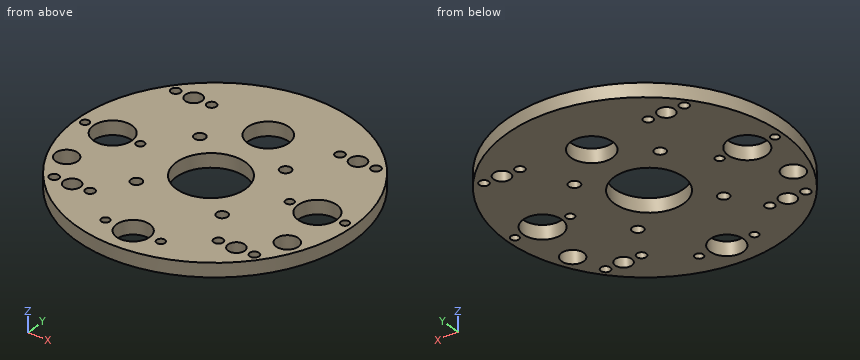
```python
from build123d import *

# Parameters (mm, degrees)
SKETCH1_R                  = 50
BOSS_EXTRUDE1_DEPTH        = 5
F_14_0_14_DIAMETER_HOLE1_D = 14
SKETCH9_R                  = 7.5
CUT_EXTRUDE1_DEPTH         = 10
SKETCH10_R                 = 12.5
SKETCH10_R_2               = 2
CUT_EXTRUDE2_DEPTH         = 10
SKETCH11_R                 = 3
CUT_EXTRUDE3_DEPTH         = 10
CIRPATTERN1_COUNT          = 4
SKETCH12_R                 = 1.5
SKETCH12_R_2               = 6
CUT_EXTRUDE4_DEPTH         = 10
SKETCH13_R                 = 4
CUT_EXTRUDE5_DEPTH         = 10
M3_CLEARANCE_HOLE1_D       = 3.4
MIRROR2_COPY_1_D           = 3.4


with BuildPart() as part:
    # Sketch1 → Boss-Extrude1 (new body)
    with BuildSketch(Plane.XY):
        Circle(SKETCH1_R)
    extrude(amount=BOSS_EXTRUDE1_DEPTH)

    # Ø14.0 (14) Diameter Hole1 (through all)
    with Locations(Plane(origin=(0, 0, 0), x_dir=(-1, 0, 0), z_dir=(0, 0, -1))):
        with Locations((37, 0), (-37, 0)):
            Hole(F_14_0_14_DIAMETER_HOLE1_D / 2)

    # Sketch9 → Cut-Extrude1 (cut)
    with BuildSketch(Plane.XY.offset(5)):
        with Locations((0, 26)):
            Circle(SKETCH9_R)
    extrude(amount=-CUT_EXTRUDE1_DEPTH, mode=Mode.SUBTRACT)

    # Sketch10 → Cut-Extrude2 (cut)
    with BuildSketch(Plane.XY.offset(5)):
        with Locations((0, -2)):
            Circle(SKETCH10_R)
        with Locations((-15.5, 13.5)):
            Circle(SKETCH10_R_2)
        with Locations((15.5, 13.5)):
            Circle(SKETCH10_R_2)
        with Locations((15.5, -17.5)):
            Circle(SKETCH10_R_2)
        with Locations((-15.5, -17.5)):
            Circle(SKETCH10_R_2)
    extrude(amount=-CUT_EXTRUDE2_DEPTH, mode=Mode.SUBTRACT)

    # Sketch11 → Cut-Extrude3 (cut)
    with BuildSketch(Plane.XY.offset(5)):
        with Locations((-29.69848481, 29.69848481)):
            Circle(SKETCH11_R)
    cut_extrude3 = extrude(amount=-CUT_EXTRUDE3_DEPTH, mode=Mode.SUBTRACT)

    # CirPattern1: Cut-Extrude3 ×4 about axis
    cirpattern1_axis = Axis((0, 0, 0), (0, 0, 1))
    for i in range(1, CIRPATTERN1_COUNT):
        add(cut_extrude3.rotate(cirpattern1_axis, i * 360 / CIRPATTERN1_COUNT), mode=Mode.SUBTRACT)

    # Sketch12 → Cut-Extrude4 (cut)
    with BuildSketch(Plane.XY.offset(5)):
        with Locations((-47, 0)):
            Circle(SKETCH12_R)
        with Locations((-27, 0)):
            Circle(SKETCH12_R)
        with Locations((27, 0)):
            Circle(SKETCH12_R)
        with Locations((47, 0)):
            Circle(SKETCH12_R)
        with Locations((-10, -40)):
            Circle(SKETCH12_R)
        with Locations((10, -40)):
            Circle(SKETCH12_R)
        with Locations((0, -40)):
            Circle(SKETCH12_R_2)
    extrude(amount=-CUT_EXTRUDE4_DEPTH, mode=Mode.SUBTRACT)

    # Sketch13 → Cut-Extrude5 (cut)
    with BuildSketch(Plane.XY.offset(5)):
        with Locations((-39.87754263, -18.595203517)):
            Circle(SKETCH13_R)
        with Locations((39.87754263, -18.595203517)):
            Circle(SKETCH13_R)
    extrude(amount=-CUT_EXTRUDE5_DEPTH, mode=Mode.SUBTRACT)

    # M3 Clearance Hole1 (through all)
    with Locations(Plane.XY.offset(5)):
        with Locations((-36.19848481, -29.69848481), (-23.19848481, -29.69848481)):
            m3_clearance_hole1 = Hole(M3_CLEARANCE_HOLE1_D / 2)

    # Mirror1: M3 Clearance Hole1 across plane
    add(m3_clearance_hole1.mirror(Plane.ZX), mode=Mode.SUBTRACT)

    # Mirror2: M3 Clearance Hole1 across plane
    add(m3_clearance_hole1.mirror(Plane(origin=(0, 0, 0), x_dir=(0, 0, 1), z_dir=(1, 0, 0))), mode=Mode.SUBTRACT)

    # Mirror2 copy 1 (through all)
    with Locations(Plane(origin=(0, 0, 5), x_dir=(-1, 0, 0), z_dir=(0, 0, 1))):
        with Locations((-36.19848481, -29.69848481), (-23.19848481, -29.69848481)):
            Hole(MIRROR2_COPY_1_D / 2)


solid = part.part
```
Here's how the part is built. I have some questions about the finished solid (model axes, mm). Coordinates: 2 decimals unless noted, no trailing zeros. Order: outer loops, then holes, each group sorted by start corner. A loop starts at its lowest first (then second) coordinate and runs counter-clockwise, first axis right, second up.
1) Imagine slicing it at A-A on y = -40. List the corners of the cut face in (x, z) for me.
2) I need wall thicknesses on line 1 (Y direction, x = -10, z = 3.9); line 2 (Y direction, x = 4, z = 4.85); line 3 (Y direction, x = -15.5, z = 1.85). Which ranges of each line are inside material? Lowest first, please.
3) Imagine slicing it at D-D on y = -12.5. List the corners of the cut face in (x, z) for me.
4) Imagine slicing it at C-C on z = 1. State how many separate pieces and enclosed holes the cut face has, and give its area (3 significant figures).
5) Imagine slicing it at B-B on x = -10. List the corners of the cut face in (y, z) for me, and give its area (3 significant figures).
6) Will these pins go through, and if not, where does the flat tip stop? pin 1 (2 mm diameter, centred on y = -39.5, z = 1, fed in from -X); pin 2 (1.5 mm diameter, centred on y = 3, z = 2.5, fed in from -X); pin 3 (1 mm diameter, centred on y = -28, z = 0.5, fed in from +X).
Response values:
1. outline: (-30, 0) - (-11.5, 0) - (-11.5, 5) - (-30, 5) - close; (-8.5, 0) - (-6, 0) - (-6, 5) - (-8.5, 5) - close; (6, 0) - (8.5, 0) - (8.5, 5) - (6, 5) - close; (11.5, 0) - (30, 0) - (30, 5) - (11.5, 5) - close
2. line 1: y = -48.99 to -41.5, -38.5 to -9.5, 5.5 to 48.99
2. line 2: y = -49.84 to -44.47, -35.53 to -13.84, 9.84 to 19.66, 32.34 to 49.84
2. line 3: y = -47.54 to -19.5, -15.5 to 11.5, 15.5 to 47.54
3. outline: (-48.41, 0) - (-6.78, 0) - (-6.78, 5) - (-48.41, 5) - close; (6.78, 0) - (48.41, 0) - (48.41, 5) - (6.78, 5) - close
4. separate pieces: 1
4. enclosed holes: 29
4. area: 6,390 mm2
5. outline: (-48.99, 0) - (-41.5, 0) - (-41.5, 5) - (-48.99, 5) - close; (-38.5, 0) - (-9.5, 0) - (-9.5, 5) - (-38.5, 5) - close; (5.5, 0) - (48.99, 0) - (48.99, 5) - (5.5, 5) - close
5. area: 400 mm2
6. pin 1: stops at x = -31.9
6. pin 2: stops at x = -49.95
6. pin 3: stops at x = 41.76
